For this review, take the finished solid that the model builds, in its own axes (mm). A direction names the side the tool comes from. Coordinates: 2 decimals unless noted, no trailing zeros. Loops run counter-clockwise (first coordinate to the right, second up) from the corner with the lowest first, then second, coordinate; pieces in that order, holes last. Notation, with made-up numbers: M 54.25,30 L 104.25,30 A23 ccw 104.25,69 Z; hole C 46,-30.5 d6. An arc over 180 degrees is marked long. Answer as a JSON object with one key per item and string values. Group by question number.
Item 1: Wall thickness on L1, parallel to X at y = 1.5, z = 0; L2, parallel to Z at x = 1.5, y = 5.5; L3, parallel to Y at x = -3.25, z = -32: over which ranges is each line inside the solid? List them lowest first. Write a range as from..to.
Item 2: Add section B-B (z = 102.5). State the section outline as (x, y) points, then the cut area to 3 significant figures.
Item 3: Tool access review of faces 1 (the face through (-2, 7, 2)), 2 (the face through (-1.915, 3.451, 4.619)): name each direction out of +Z, -Z, +X, -X, +Y, -Y from which nothing blocks a thin tool from reaching the whole face with its end or side.
Item 4: Insertion check: pin 1 (3 mm diameter, centred on x = 3, z = -93.5, fed in from +Y); pin 2 (1.5 mm diameter, centred on y = 3, z = -69.5, fed in from +X); pin 3 (4 mm diameter, centred on y = 1, z = -5.5, fed in from -X). Each pin has a flat end and moves straight along its axis. Give the tip position at first contact, or say it passes through.
Item 5: Add section A-A (z = 0). State the section outline as (x, y) points.
Item 6: Mouldability with a two-part tool opening along Z and no side actions: class faces 3 (the face through (-0.43, 4.12, 63.93)), 4 (the face through (0, 4, 127)), 5 (the face through (0, 4, -127)), 6 (the face through (-2.44, 3.55, -0.54)) as +Z half, -Z half, draft (parallel to the pull), parting line (faces both ways), or undercut.
from build123d import *

# Parameters (mm, degrees)
SKETCH_1_R               = 5
EXTRUDE_1_DEPTH          = 7
EXTRUDE_2_DEPTH          = 127
PATTERN_CIRCULAR_1_COUNT = 2
CUT_EXTRUDE_1_REACH      = 129.291
SKETCH_2_R               = 2.5


with BuildPart() as part:
    # 草图1 → 凸台-拉伸1 (new body)
    with BuildSketch(Plane(origin=(0, 0, 0), x_dir=(1, 0, 0), z_dir=(0, 1, 0))):
        with Locations(Location((0, 0, 0), (0, 0, 270))):
            Circle(SKETCH_1_R)
    extrude(amount=EXTRUDE_1_DEPTH)

    # 草图3 → 凸台-拉伸2 (add)
    with BuildSketch(Plane.XY):
        Polygon((-4.272114317, 1.899519053), (3.522114317, 6.399519053), (4.272114317, 5.100480947), (-3.522114317, 0.600480947), align=None)
    extrude_2 = extrude(amount=EXTRUDE_2_DEPTH)

    # 阵列(圆周)1: 凸台-拉伸2 ×2 about axis
    pattern_circular_1_axis = Axis((0, 0, 0), (0, 1, 0))
    for i in range(1, PATTERN_CIRCULAR_1_COUNT):
        add(extrude_2.rotate(pattern_circular_1_axis, i * 360 / PATTERN_CIRCULAR_1_COUNT))

    # 草图2 → 切除-拉伸1 (cut, up to next)
    with BuildSketch(Plane(origin=(0, 7, 0), x_dir=(1, 0, 0), z_dir=(0, 1, 0)), mode=Mode.PRIVATE) as cut_extrude_1_sk1:
        with Locations(Location((0, 0, 0), (0, 0, 270))):
            Circle(SKETCH_2_R)
    cut_extrude_1_tool1 = extrude(cut_extrude_1_sk1.sketch, amount=-CUT_EXTRUDE_1_REACH, mode=Mode.PRIVATE) & part.part
    add(cut_extrude_1_tool1.solids().sort_by_distance((0, 7, 0))[0], mode=Mode.SUBTRACT)


solid = part.part
From the geometry:
{
 "1": {"L1": "x = -5..-2.5, 2.5..5", "L2": "z = -4.77..-2, 2..4.77", "L3": "y = 4.51..6.24"},
 "2": {"outline": "M -4.27,1.9 L -3.52,0.6 L 4.27,5.1 L 3.52,6.4 Z", "area": "13.5 mm²"},
 "3": {"face 1": "+Z, -Z, +X, -X, +Y", "face 2": "none"},
 "4": {"pin 1": "stops at y = 3.5", "pin 2": "stops at x = 3.67", "pin 3": "stops at x = -3.57"},
 "5": {"outline": "M -5,0 L -2.5,0 L -2.5,7 L -5,7 Z; M 2.5,0 L 5,0 L 5,7 L 2.5,7 Z"},
 "6": {"face 3": "draft", "face 4": "+Z half", "face 5": "-Z half", "face 6": "undercut"}
}
